Source: CAD feature listing. Evaluate the final solid. Frame: model axes, mm. Face numbers are marked on the shaded views. A direction names the side the tool comes from. Coordinates: 2 decimals unless noted, no trailing zeros. Order: outer loops, then holes, each group sorted by start corner. A loop starts at its lowest first (then second) coordinate and runs counter-clockwise, first axis right, second up.
Item 1: Mould query, pull axis X, two halves, no side actions, for the marked faces 1, 2 and 3. Classes: released by +X, released by -X, zero draft, split by the parting line, or undercut.
Item 2: Ray query, line 1 (Y direction, x = 171.5, z = -63.5); line 2 (X direction, y = 67.5, z = -104.5); line 3 (Z direction, x = 174.75, y = 50.8). Return the intervals inside material, ascending.
Item 3: Section D-D on y = 50.8. Return the cut outline in (x, z), then the cut area to 3 significant figures.
Item 4: Section B-B on x = 25.4. Return the cut outline in (y, z) (3 decimals).
Item 5: Contact query for flat-ended pins moving along their axis: P1, Ø4, axis at y = 65, z = -19.5, coming from the +X side; P2, Ø12, axis at x = 194, z = -83.5, coming from the +Y side. Output: stop coordinate, or through.
Item 6: Section A-A on y = 91.5. Return the cut outline in (x, z), then the cut area to 3 significant figures.
Item 7: Reachability of the marked faces 4, 5, 6 and 7 from +Z, -Z, +X, -X, +Y, -Y: full face, straight path, thin tool, end or side. Return the list, or none.
Item 8: Section C-C on z = -63.5. Return the cut outline in (x, y) (3 decimals).
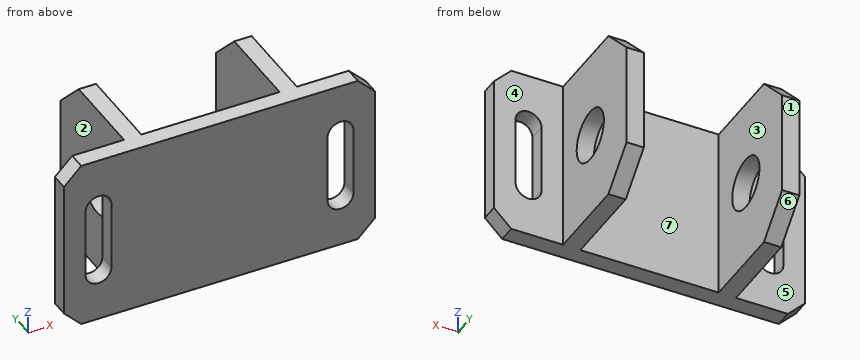
Autodesk Inventor part; units mm, degrees
ref_plane "Work Plane1" through (114.3, 0, -114.3) normal (-1, 0, 0) x (0, 0, 1)
ref_plane "YZ Plane" through (0, 0, 0) normal (1, 0, 0) x (0, 1, 0)
ref_plane "XZ Plane" through (0, 0, 0) normal (0, 1, 0) x (-1, 0, 0)
sketch "Sketch1" plane through (0, 0, 0) normal (0, 1, 0) x (-1, 0, 0)
  line L0 (0, 0) -> (-228.6, 0)
  line L1 (-228.6, 0) -> (-228.6, -127)
  line L2 (-228.6, -127) -> (0, -127)
  line L3 (0, -127) -> (0, 0)
  dimension "d0" = 228.6
  dimension "d1" = 127
extrude "Extrusion1" add sketch "Sketch1" along normal blind 12.7
chamfer "Chamfer1" distance 12.7 angle 45 4 edges at (0, 6.35, 0) (228.6, 6.35, 0) (228.6, 6.35, -127) (0, 6.35, -127)
sketch "Sketch2" plane through (0, 12.7, 0) normal (0, 1, 0) x (1, 0, 0)
  line L0 (12.7, 0) -> (215.9, 0)
  line L1 (114.3, 0) -> (63.5, 0)
  line L2 (63.5, 0) -> (63.5, 127)
  line L3 (63.5, 127) -> (114.3, 127)
  line L4 (114.3, 127) -> (114.3, 0)
  line L5 (215.9, 127) -> (12.7, 127)
  line L6 (63.5, 0) -> (50.8, 0)
  line L7 (50.8, 0) -> (50.8, 127)
  line L8 (50.8, 127) -> (63.5, 127)
  line L9 (63.5, 127) -> (63.5, 0)
  line L10 (114.3, 0) -> (165.1, 0)
  line L11 (165.1, 0) -> (165.1, 127)
  line L12 (165.1, 127) -> (114.3, 127)
  line L13 (114.3, 127) -> (114.3, 0)
  line L14 (165.1, 0) -> (177.8, 0)
  line L15 (177.8, 0) -> (177.8, 127)
  line L16 (177.8, 127) -> (165.1, 127)
  line L17 (165.1, 127) -> (165.1, 0)
  point P0 (0, 0)
  dimension "d7" = 50.8
  dimension "d8" = 127
  dimension "d9" = 12.7
  dimension "d10" = 50.8
  dimension "d11" = 12.7
extrude "Extrusion2" add sketch "Sketch2" along normal blind 88.9 contours L7 L5 L2 L0 | L11 L5 L15 L0
chamfer "Chamfer2" distance 25.4 angle 45 4 edges at (57.15, 101.6, 0) (57.15, 101.6, -127) (171.45, 101.6, 0) (171.45, 101.6, -127)
sketch "Sketch3" plane through (177.8, 12.7, 0) normal (1, 0, 0) x (0, 0, -1)
  line L0 (0, 0) -> (0, 63.5)
  line L1 (127, 0) -> (127, 63.5)
  line L2 (101.6, 88.9) -> (25.4, 88.9)
  line L3 (63.5, 88.9) -> (63.5, 38.1)
  circle A0 centre (63.5, 38.1) radius 19.05
  point P0 (0, -12.7)
  dimension "d17" = 50.8
  dimension "d18" = 38.1
extrude "Extrusion3" cut sketch "Sketch3" against normal through all
sketch "Sketch6" plane through (0, 12.7, 0) normal (0, 1, 0) x (1, 0, 0)
  arc A0 (207.9625, 88.9) -> (198.4375, 88.9) centre (203.2, 88.9) ccw
  circle A1 centre (203.2, 88.9) radius 9.525
  arc A2 (198.4375, 38.1) -> (207.9625, 38.1) centre (203.2, 38.1) ccw
  circle A3 centre (203.2, 38.1) radius 9.525
  line L0 (193.675, 38.1) -> (193.675, 88.9)
  line L1 (212.725, 38.1) -> (212.725, 88.9)
  point P0 (0, 0)
  dimension "d31" = 19.05
  dimension "d32" = 19.05
extrude "Extrusion5" cut sketch "Sketch6" against normal blind 25.4
ref_plane "Work Plane1" through (114.3, 0, -114.3) normal (-1, 0, 0) x (0, 0, 1)
mirror "Mirror1" about plane through (114.3, 0, -114.3) normal (-1, 0, 0) of "Extrusion5"
properties part number "Block3" material "Aluminum 6061"
Answer list:
1. face 1: zero draft
1. face 2: released by -X
1. face 3: undercut
2. line 1: y = 0 to 31.75, 69.85 to 101.6
2. line 2: x = 50.8 to 63.5, 165.1 to 177.8
2. line 3: z = -127 to -82.55, -44.45 to 0
3. outline: (50.8, -127) - (63.5, -127) - (63.5, -82.55) - (50.8, -82.55) - close; (50.8, -44.45) - (63.5, -44.45) - (63.5, 0) - (50.8, 0) - close; (165.1, -127) - (177.8, -127) - (177.8, -82.55) - (165.1, -82.55) - close; (165.1, -44.45) - (177.8, -44.45) - (177.8, 0) - (165.1, 0) - close
3. area: 2,260 mm2
4. outline: (0, -127) - (12.7, -127) - (12.7, -98.425) - (0, -98.425) - close; (0, -28.575) - (12.7, -28.575) - (12.7, 0) - (0, 0) - close
5. P1: stops at x = 177.8
5. P2: stops at y = 12.7
6. outline: (50.8, -111.7) - (63.5, -111.7) - (63.5, -15.3) - (50.8, -15.3) - close; (165.1, -111.7) - (177.8, -111.7) - (177.8, -15.3) - (165.1, -15.3) - close
6. area: 2,450 mm2
7. face 4: +Z, -Z, +X, +Y
7. face 5: +Z, -Z, -X, +Y
7. face 6: -Z, +X, -X, +Y
7. face 7: +Z, -Z, +Y
8. outline: (0, 0) - (15.875, 0) - (15.875, 12.7) - (0, 12.7) - close; (34.925, 0) - (193.675, 0) - (193.675, 12.7) - (177.8, 12.7) - (177.8, 31.75) - (165.1, 31.75) - (165.1, 12.7) - (63.5, 12.7) - (63.5, 31.75) - (50.8, 31.75) - (50.8, 12.7) - (34.925, 12.7) - close; (50.8, 69.85) - (63.5, 69.85) - (63.5, 101.6) - (50.8, 101.6) - close; (165.1, 69.85) - (177.8, 69.85) - (177.8, 101.6) - (165.1, 101.6) - close; (212.725, 0) - (228.6, 0) - (228.6, 12.7) - (212.725, 12.7) - close
